Here's how the part is built. I have some questions about the finished solid (model axes, mm). A direction names the side the tool comes from. Coordinates: 2 decimals unless noted, no trailing zeros. Write each loop counter-clockwise with the first axis right and the second up, starting at its lowest first coordinate (ties: lowest second). Pieces come first, ordered by that corner, then holes. Notation, with made-up numbers: (46, 89.25) -> (70, 89.25) arc R15 cw to (70, 99.25) -> close; hole circle Ø2 at (-32.75, -17.5). An arc over 180 degrees is marked (long way). Use a Markdown table: item, result. Add a question column.
Item 1: On a 3-axis mill with a long thin cutter (end or side, diameter ignored), from which of +Z, -Z, +X, -X, +Y, -Y can I reach the whole of each face in a straight line? I mean faces 1 (the flat face through (18.787, 27, 15)), 2 (the flat face through (23, -0.394, 15)), 3 (the flat face through (-1, 9, 7)), 4 (the flat face through (-0.3, 33.106, 6.8)), 5 (the flat face through (16.787, -8, 15)). Say none if no direction works.
Item 2: Imagine slicing it at C-C, the plane x = 6. Write out the boundary of the cut face in (y, z).
Item 3: Will these pins go through, and if not, where does the flat tip stop? pin 1 Ø11.5 at (y, z) = (-10, 16.5) entering from +X; pin 2 Ø8 at (y, z) = (4, 22.5) entering from -X; pin 3 Ø8.5 at (x, z) = (26.5, 18) entering from -Y.
Item 4: If I drill on line 1 along X through (y, z) = (-2, 8.25); line 2 along Z through (x, y) = (-22, 4); line 3 along Y through (x, z) = (20.5, 11.5), over which ranges is the centre line in solid material (lowest first)? Write a range as from..to.
Item 5: Imagine slicing it at D-D, the plane y = 29.5. Write out the boundary of the cut face in (x, z), and give its area (3 significant figures).
Item 6: If we mould it in two halves opening along Y, with no side actions, what happens to faces 6 (the cylindrical face through (-17.68, 19.13, 23.19)), 7 (the flat face through (-1, 39.106, 2)), 8 (the flat face through (-1, -17, 5))? For each: pulls with the +Y half, pulls with the -Y half, needs draft (parallel to the pull), parting line crosses it, or undercut.
Item 7: Imagine slicing it at B-B, the plane y = 12. Write out the boundary of the cut face in (x, z).
Item 8: Imagine slicing it at A-A, the plane z = 18.25. Count the separate pieces of the cut face and the enclosed holes in it, and give its area (3 significant figures).
```python
from build123d import *

# Parameters (mm, degrees)
SKETCH1_W           = 78
SKETCH1_H           = 60
BOSS_EXTRUDE1_DEPTH = 5
SKETCH7_R           = 3
CUT_EXTRUDE4_DEPTH  = 56.605062255
SKETCH8_W           = 38
SKETCH8_H           = 48
BOSS_EXTRUDE2_DEPTH = 20
SKETCH9_W           = 58.87856647
SKETCH9_H           = 23
BOSS_EXTRUDE3_DEPTH = 20
SKETCH10_W          = 16
SKETCH10_H          = 19
CUT_EXTRUDE5_DEPTH  = 60
SKETCH11_W          = 34
SKETCH11_H          = 16
CUT_EXTRUDE6_DEPTH  = 60
SKETCH12_R          = 2.5
CUT_EXTRUDE7_DEPTH  = 9


with BuildPart() as part:
    # Sketch1 → Boss-Extrude1 (new body)
    with BuildSketch(Plane.XY):
        with Locations((-0.21253406, 9.10626703)):
            Rectangle(SKETCH1_W, SKETCH1_H)
    extrude(amount=BOSS_EXTRUDE1_DEPTH)

    # Sketch7 → Cut-Extrude4 (cut, through all)
    with BuildSketch(Plane.XY.offset(5)):
        with Locations((-23.21253406, 24.10626703)):
            Circle(SKETCH7_R)
        with Locations((22.78746594, 24.10626703)):
            Circle(SKETCH7_R)
        with Locations((22.78746594, -5.89373297)):
            Circle(SKETCH7_R)
        with Locations((-23.21253406, -5.89373297)):
            Circle(SKETCH7_R)
    extrude(amount=-CUT_EXTRUDE4_DEPTH, mode=Mode.SUBTRACT)

    # Sketch8 → Boss-Extrude2 (add)
    with BuildSketch(Plane.XY.offset(5)):
        with Locations((-0.21253406, 9.10626703)):
            Rectangle(SKETCH8_W, SKETCH8_H)
    extrude(amount=BOSS_EXTRUDE2_DEPTH)

    # Sketch9 → Boss-Extrude3 (add)
    with BuildSketch(Plane.XY.offset(5)):
        with Locations((-0.21253406, 9.10626703)):
            Rectangle(SKETCH9_W, SKETCH9_H)
    extrude(amount=BOSS_EXTRUDE3_DEPTH)

    # Sketch10 → Cut-Extrude5 (cut)
    with BuildSketch(Plane.ZY.offset(29.651817295)):
        with Locations((15, 9.10626703)):
            Rectangle(SKETCH10_W, SKETCH10_H)
    extrude(amount=-CUT_EXTRUDE5_DEPTH, mode=Mode.SUBTRACT)

    # Sketch11 → Cut-Extrude6 (cut)
    with BuildSketch(Plane.XZ.offset(14.89373297)):
        with Locations((-0.21253406, 15)):
            Rectangle(SKETCH11_W, SKETCH11_H)
    extrude(amount=-CUT_EXTRUDE6_DEPTH, mode=Mode.SUBTRACT)

    # Sketch12 → Cut-Extrude7 (cut)
    with BuildSketch(Plane.XY.offset(25)):
        with Locations((-16.211721725, 17.10626703)):
            Circle(SKETCH12_R)
        with Locations((14.788278275, 17.10626703)):
            Circle(SKETCH12_R)
    extrude(amount=-CUT_EXTRUDE7_DEPTH, mode=Mode.SUBTRACT)


solid = part.part
```
Ans:
| question | item | result |
|---|---|---|
| 1 | face 1 | +Z, +X, +Y |
| 1 | face 2 | +X, -X |
| 1 | face 3 | none |
| 1 | face 4 | +Z, +X, -X, +Y |
| 1 | face 5 | +Y, -Y |
| 2 | outline | (-20.89, 0) -> (39.11, 0) -> (39.11, 5) -> (33.11, 5) -> (33.11, 7) -> (-14.89, 7) -> (-14.89, 5) -> (-20.89, 5) -> close; (-14.89, 23) -> (33.11, 23) -> (33.11, 25) -> (-14.89, 25) -> close |
| 3 | pin 1 | stops at x = 18.79 |
| 3 | pin 2 | stops at x = -29.65 |
| 3 | pin 3 | stops at y = -2.39 |
| 4 | line 1 | x = -29.65..-17.21, 16.79..29.23 |
| 4 | line 2 | z = 0..7, 23..25 |
| 4 | line 3 | y = -2.39..-0.39, 18.61..20.61 |
| 5 | outline | (-39.21, 0) -> (38.79, 0) -> (38.79, 5) -> (18.79, 5) -> (18.79, 25) -> (-19.21, 25) -> (-19.21, 5) -> (-39.21, 5) -> close; hole (-17.21, 7) -> (16.79, 7) -> (16.79, 23) -> (-17.21, 23) -> close |
| 5 | area | 606 mm^2 |
| 6 | face 6 | undercut |
| 6 | face 7 | pulls with the +Y half |
| 6 | face 8 | needs draft |
| 7 | outline | (-39.21, 0) -> (38.79, 0) -> (38.79, 5) -> (29.23, 5) -> (29.23, 7) -> (-29.65, 7) -> (-29.65, 5) -> (-39.21, 5) -> close; (-29.65, 23) -> (29.23, 23) -> (29.23, 25) -> (-29.65, 25) -> close |
| 8 | separate pieces | 4 |
| 8 | enclosed holes | 0 |
| 8 | area | 199 mm^2 |
